Design review of the part built by this model. Coordinates are the model's own, in mm. Face numbers are marked on the shaded views. A direction names the side the tool comes from. Round coordinates to 2 decimals unless told otherwise and drop trailing zeros. Order: outer loops, then holes, each group sorted by start corner. A loop starts at its lowest first (then second) coordinate and runs counter-clockwise, first axis right, second up.
Autodesk Inventor part; units mm, degrees
ref_plane "YZ Plane" through (0, 0, 0) normal (1, 0, 0) x (0, 1, 0)
ref_plane "XZ Plane" through (0, 0, 0) normal (0, 1, 0) x (-1, 0, 0)
ref_plane "XY Plane" through (0, 0, 0) normal (0, 0, 1) x (1, 0, 0)
sketch "Sketch1" plane through (0, 0, 0) normal (0, 0, 1) x (1, 0, 0)
  line L0 (3.175, 17) -> (4.5761, 13.6173)
  line L1 (6.4239, 13.6173) -> (7.825, 17)
  arc A0 (4.5761, 13.6173) -> (6.4239, 13.6173) centre (5.5, 14) ccw
  line L2 (7.825, 17) -> (9, 17)
  line L3 (3.175, 17) -> (0, 17)
  line L4 (2, 11) -> (9, 11)
  line L5 (9, 17) -> (9, 11)
  line L6 (0, 17) -> (0, 8.5)
  line L7 (2, 11) -> (2, 8.5)
  line L8 (2, 8.5) -> (0, 8.5)
  line L9 (0, 0) -> (2, 0) construction
  point P0 (5.5, 11)
  dimension "d0" = 45
  dimension "d1" = 1
  dimension "d2" = 3
  dimension "d4" = 6
  dimension "d5" = 2
  dimension "d8" = 7
  dimension "d9" = 17
  dimension "d10" = 22
revolve "Revolution1" add sketch "Sketch1" angle 360 about axis through (0, 0, 0) along (1, 0, 0)
sketch "Sketch2" plane through (9, 0, 0) normal (1, 0, 0) x (0, 0, -1)
  circle A0 centre (0, 0) radius 11
  circle A1 centre (0, 0) radius 17
  line L0 (-17, 0) -> (17, 0) construction
  line L1 (-12.0208, -12.0208) -> (12.0208, 12.0208) construction
  line L2 (0, -17) -> (0, 17) construction
  line L3 (12.0208, -12.0208) -> (-12.0208, 12.0208) construction
  line L4 (-17, 0) -> (-11, 0)
  line L5 (-7.7782, 7.7782) -> (-12.0208, 12.0208)
  line L6 (0, 17) -> (0, 11)
  line L7 (12.0208, 12.0208) -> (7.7782, 7.7782)
  line L8 (11, 0) -> (17, 0)
  line L9 (12.0208, -12.0208) -> (7.7782, -7.7782)
  line L10 (0, -17) -> (0, -11)
  line L11 (-7.7782, -7.7782) -> (-12.0208, -12.0208)
  arc A2 (7.7782, 7.7782) -> (0, 11) centre (0, 0) ccw
  arc A3 (12.0208, 12.0208) -> (0, 17) centre (0, 0) ccw
  arc A4 (7.7782, -7.7782) -> (11, 0) centre (0, 0) ccw
  arc A5 (12.0208, -12.0208) -> (17, 0) centre (0, 0) ccw
  arc A6 (-12.0208, 12.0208) -> (-17, 0) centre (0, 0) ccw
  arc A7 (-12.0208, -12.0208) -> (0, -17) centre (0, 0) ccw
  arc A8 (-7.7782, 7.7782) -> (-11, 0) centre (0, 0) ccw
  arc A9 (-7.7782, -7.7782) -> (0, -11) centre (0, 0) ccw
  dimension "d14" = 135
extrude "Extrusion1" cut sketch "Sketch2" against normal blind 4.424 contours L8 A1 L9 A0 | A0 L6 A1 L7 | L10 A1 L11 A0 | A0 L4 A1 L5
sketch "Sketch3" plane through (9, 0, 17) normal (1, 0, 0) x (0, 0, -1)
  line L0 (4.9792, -12.0208) -> (9.2218, -7.7782)
  arc A0 (6, 0) -> (9.2218, -7.7782) centre (17, 0) ccw
  line L1 (6, 0) -> (0, 0)
  arc A1 (0, 0) -> (4.9792, -12.0208) centre (17, 0) ccw
  line L2 (4.9792, 12.0208) -> (9.2218, 7.7782)
  arc A2 (17, 11) -> (9.2218, 7.7782) centre (17, 0) ccw
  line L3 (17, 11) -> (17, 17)
  arc A3 (17, 17) -> (4.9792, 12.0208) centre (17, 0) ccw
  line L4 (28, 0) -> (34, 0)
  arc A4 (34, 0) -> (29.0208, 12.0208) centre (17, 0) ccw
  line L5 (29.0208, 12.0208) -> (24.7782, 7.7782)
  arc A5 (28, 0) -> (24.7782, 7.7782) centre (17, 0) ccw
  line L6 (17, -11) -> (17, -17)
  arc A6 (17, -17) -> (29.0208, -12.0208) centre (17, 0) ccw
  line L7 (29.0208, -12.0208) -> (24.7782, -7.7782)
  arc A7 (17, -11) -> (24.7782, -7.7782) centre (17, 0) ccw
extrude "Extrusion2" cut sketch "Sketch3" against normal blind 2.424
chamfer "Chamfer1" distance 1 angle 45 1 edges at (0, -17, 0)
properties part number "rope_pulley" material "ABS Plastic"
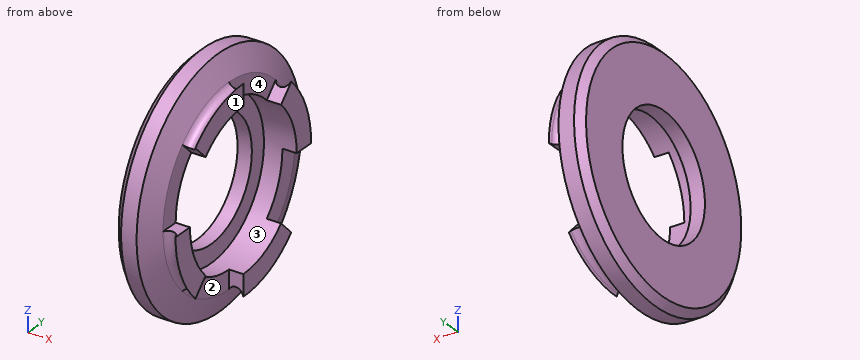
1) Take a section at A-A on x = 6. Give the boundary of the cut face in (y, z), plus the area to 3 significant figures.
Results:
outline: (-13.13, 0) arc R13.13 ccw to (-9.29, -9.29) - (-7.78, -7.78) arc R11 cw to (-11, 0) - close; (-9.29, 9.29) - (-7.78, 7.78) arc R11 cw to (0, 11) - (0, 13.13) arc R13.13 ccw to start; (0, -13.13) arc R13.13 ccw to (9.29, -9.29) - (7.78, -7.78) arc R11 cw to (0, -11) - close; (7.78, 7.78) arc R11 cw to (11, 0) - (13.13, 0) arc R13.13 ccw to (9.29, 9.29) - close
area: 80.9 mm2
2) For the marked faces 1, 2, 3 and 4, list the 3-axis set-ups (+Z, -Z, +X, -X, +Y, -Y) from which the entire face can be reached by the end or side of a thin tool; tool diameter is ignored.
Results:
face 1: +Z, -Z, +X, +Y, -Y
face 2: -Z, +X
face 3: +X
face 4: +Z, +X
3) Clearance check with flat-ended pins moving along their axes: P1, Ø13, axis at y = 0, z = 0, coming from the -X side; P2, Ø2, axis at x = 3, y = -13, coming from the -Z side; P3, Ø10, axis at y = -0.5, z = -5, coming from the +X side; P4, Ø2, axis at x = 4, z = -4, coming from the -Y side. State where each tip first meets the part, or that it passes through.
Results:
P1: passes through
P2: stops at z = -12.04
P3: stops at x = 2
P4: stops at y = -16.65
4) To check wall thickness, follow line 1 along Z through (x, y) = (1.45, 0); line 2 along X through (y, z) = (6, -9); line 3 along Z through (x, y) = (3, -10). State the ranges of each line that lie inside material, in increasing order.
Results:
line 1: z = -17 to -8.5, 8.5 to 17
line 2: x = 0 to 2
line 3: z = -13.75 to -4.58, 4.58 to 13.75
